```python
from build123d import *

# Parameters (mm, degrees)
BOSS_EXTRUDE1_DEPTH     = 15.24
SKETCH3_R               = 2.5
BOSS_EXTRUDE2_DEPTH     = 2.54
SKETCH4_W               = 6.457620629
SKETCH4_H               = 27.913585942
BOSS_EXTRUDE3_DEPTH     = 7.62
SKETCH11_W              = 6.457620629
SKETCH11_H              = 27.913585942
BOSS_EXTRUDE6_DEPTH     = 2.0955
CUT_EXTRUDE1_DEPTH      = 111.34392643
CUT_EXTRUDE1_DEPTH_BACK = 3.332
SKETCH6_R               = 2.15
FILLET1_R               = 0.508
SKETCH8_W               = 21.59
SKETCH8_H               = 20.32
CUT_EXTRUDE2_DEPTH      = 111.477226273
SKETCH1_3_W             = 10
SKETCH1_3_H             = 13.208
SKETCH1_3_R             = 2
BOSS_EXTRUDE5_DEPTH     = 2.54
CUT_EXTRUDE5_DEPTH      = 9.2075
CUT_EXTRUDE5_DEPTH_BACK = 117.302117887
SKETCH14_W              = 50.8
SKETCH14_H              = 3.81
BOSS_EXTRUDE7_START     = -7.62
SKETCH15_W              = 5.08
SKETCH15_H              = 5.08
SKETCH15_H_2            = 8.89
BOSS_EXTRUDE7_DEPTH     = 7.62
CUT_EXTRUDE6_REACH      = 118.302
SKETCH16_R              = 1.0922
SKETCH18_W              = 22.782868823
SKETCH18_H              = 5.08
BOSS_EXTRUDE8_DEPTH     = 5.08
CUT_EXTRUDE3_DEPTH      = 12.7
CUT_EXTRUDE3_DEPTH_BACK = 12.7
SKETCH9_R               = 1.4986
SKETCH10_R              = 2.794
CUT_EXTRUDE4_DEPTH      = 2
SKETCH20_R              = 2.15
BOSS_EXTRUDE9_DEPTH     = 1
BOSS_EXTRUDE10_START    = -1
SKETCH21_R              = 2.15
BOSS_EXTRUDE10_DEPTH    = 1


with BuildPart() as part:
    # Sketch1 → Boss-Extrude1 (new body)
    with BuildSketch(Plane(origin=(0, 0, 0), x_dir=(1, 0, 0), z_dir=(0, 1, 0))):
        Polygon((-58.867621619, 16.51), (-58.867621619, -16.51), (96.852680324, -16.51), (96.852680324, -11.43), (55.88, -11.43), (55.88, 8.89), (106.68, 8.89), (106.68, 16.51), align=None)
    extrude(amount=BOSS_EXTRUDE1_DEPTH)

    # Sketch3 → Boss-Extrude2 (add)
    with BuildSketch(Plane.XY.offset(16.51)):
        with BuildLine():
            Line((4.445, 15.24), (-4.445, 15.24))
            Line((-4.445, 15.24), (-4.445, 34.29))
            ThreePointArc((-4.445, 34.29), (0, 38.735), (4.445, 34.29))
            Line((4.445, 34.29), (4.445, 15.24))
        make_face()
        with Locations((0, 34.29)):
            Circle(SKETCH3_R, mode=Mode.SUBTRACT)
    boss_extrude2 = extrude(amount=-BOSS_EXTRUDE2_DEPTH)

    # Mirror1: Boss-Extrude2 across plane
    add(boss_extrude2.mirror(Plane.XY))

    # Sketch4 → Boss-Extrude3 (add)
    with BuildSketch(Plane(origin=(0, 15.24, 0), x_dir=(1, 0, 0), z_dir=(0, 1, 0))):
        with Locations((29.475913514, 0)):
            Rectangle(SKETCH4_W, SKETCH4_H)
        with Locations((-29.475913514, 0)):
            Rectangle(SKETCH4_W, SKETCH4_H)
    extrude(amount=BOSS_EXTRUDE3_DEPTH)

    # Sketch11 → Boss-Extrude6 (add)
    with BuildSketch(Plane(origin=(0, 22.86, 0), x_dir=(1, 0, 0), z_dir=(0, 1, 0))):
        with Locations((29.475913514, 0)):
            Rectangle(SKETCH11_W, SKETCH11_H)
    extrude(amount=BOSS_EXTRUDE6_DEPTH)

    # Sketch6 → Cut-Extrude1 (cut, two sides: drawn at the far end of the back side and taken through both)
    with BuildSketch(Plane(origin=(0, 22.86, 0), x_dir=(1, 0, 0), z_dir=(0, 1, 0)).offset(-CUT_EXTRUDE1_DEPTH_BACK)):
        with Locations(Location((29.5986053, 8.550450758, 0), (0, 0, 270))):
            Circle(SKETCH6_R)
        with Locations(Location((29.5986053, -8.550450758, 0), (0, 0, 270))):
            Circle(SKETCH6_R)
        with Locations(Location((-29.5986053, -8.550450758, 0), (0, 0, 90))):
            Circle(SKETCH6_R)
        with Locations(Location((-29.5986053, 8.550450758, 0), (0, 0, 90))):
            Circle(SKETCH6_R)
    extrude(amount=CUT_EXTRUDE1_DEPTH + CUT_EXTRUDE1_DEPTH_BACK, mode=Mode.SUBTRACT)

    # Fillet1
    fillet1_edges = [part.edges().sort_by_distance(p)[0] for p in [
        (-58.867621619, 0, 0),
        (106.68, 0, -12.7),
        (18.992529352, 0, 16.51),
        (-58.867621619, 7.62, 16.51),
        (-58.867621619, 7.62, -16.51),
        (106.68, 7.62, -16.51),
        (106.68, 7.62, -8.89),
        (96.852680324, 7.62, 16.51),
        (106.68, 15.24, -12.7),
        (-58.867621619, 15.24, 0),
        (-26.247103199, 22.86, 0),
        (-29.475913514, 22.86, -13.956792971),
        (-32.704723828, 22.86, 0),
        (-29.475913514, 22.86, 13.956792971),
        (32.704723828, 24.9555, 0),
        (29.475913514, 24.9555, -13.956792971),
        (26.247103199, 24.9555, 0),
        (29.475913514, 24.9555, 13.956792971),
    ]]
    fillet(fillet1_edges, radius=FILLET1_R)

    # Sketch8 → Cut-Extrude2 (cut, through all)
    with BuildSketch(Plane(origin=(0, 15.24, 0), x_dir=(1, 0, 0), z_dir=(0, 1, 0))):
        with Locations((46.028773367, -1.27)):
            Rectangle(SKETCH8_W, SKETCH8_H)
    extrude(amount=-CUT_EXTRUDE2_DEPTH, mode=Mode.SUBTRACT)

    # Sketch1<3> → Boss-Extrude5 (add)
    # profile 1 of 2: a face of its own
    with BuildSketch(Plane(origin=(0, 0, 0), x_dir=(1, 0, 0), z_dir=(0, 1, 0))):
        with Locations((-41.488351659, 23.114)):
            Rectangle(SKETCH1_3_W, SKETCH1_3_H)
        with Locations(Location((-41.488351659, 20.01, 0), (0, 0, 270))):
            Circle(SKETCH1_3_R, mode=Mode.SUBTRACT)
    # profile 2 of 2: a face of its own
    with BuildSketch(Plane(origin=(0, 0, 0), x_dir=(1, 0, 0), z_dir=(0, 1, 0))):
        with Locations((41.488351659, 23.114)):
            Rectangle(SKETCH1_3_W, SKETCH1_3_H)
        with Locations(Location((41.488351659, 20.01, 0), (0, 0, 270))):
            Circle(SKETCH1_3_R, mode=Mode.SUBTRACT)
    extrude(amount=BOSS_EXTRUDE5_DEPTH)

    # Sketch14 → Cut-Extrude5 (cut, two sides: drawn at the far end of the back side and taken through both)
    with BuildSketch(Plane.XY.offset(-8.89).offset(-CUT_EXTRUDE5_DEPTH_BACK)):
        with Locations((81.28, 13.335)):
            Rectangle(SKETCH14_W, SKETCH14_H)
    extrude(amount=CUT_EXTRUDE5_DEPTH + CUT_EXTRUDE5_DEPTH_BACK, mode=Mode.SUBTRACT)

    # Sketch15 → Boss-Extrude7 (add)
    with BuildSketch(Plane.XY.offset(-8.89).offset(BOSS_EXTRUDE7_START)):
        with Locations((53.34, 17.78)):
            Rectangle(SKETCH15_W, SKETCH15_H)
        with Locations((82.169, 15.875)):
            Rectangle(SKETCH15_W, SKETCH15_H_2)
    extrude(amount=BOSS_EXTRUDE7_DEPTH)

    # Sketch16 → Cut-Extrude6 (cut, up to next)
    with BuildSketch(Plane.XY.offset(-8.89), mode=Mode.PRIVATE) as cut_extrude6_sk1:
        with Locations((53.34, 17.526)):
            Circle(SKETCH16_R)
    cut_extrude6_tool1 = extrude(cut_extrude6_sk1.sketch, amount=-CUT_EXTRUDE6_REACH, mode=Mode.PRIVATE) & part.part
    # Sketch16 → Cut-Extrude6 (cut, up to next)
    with BuildSketch(Plane.XY.offset(-8.89), mode=Mode.PRIVATE) as cut_extrude6_sk2:
        with Locations((81.7245, 17.526)):
            Circle(SKETCH16_R)
    cut_extrude6_tool2 = extrude(cut_extrude6_sk2.sketch, amount=-CUT_EXTRUDE6_REACH, mode=Mode.PRIVATE) & part.part
    add(cut_extrude6_tool1.solids().sort_by_distance((53.34, 17.526, -8.89))[0], mode=Mode.SUBTRACT)
    add(cut_extrude6_tool2.solids().sort_by_distance((81.7245, 17.526, -8.89))[0], mode=Mode.SUBTRACT)

    # Sketch18 → Boss-Extrude8 (add)
    with BuildSketch(Plane(origin=(0, 15.24, 0), x_dir=(1, 0, 0), z_dir=(0, 1, 0))):
        with Locations((84.032315508, -13.97)):
            Rectangle(SKETCH18_W, SKETCH18_H)
    extrude(amount=BOSS_EXTRUDE8_DEPTH)

    # Sketch9 → Cut-Extrude3 (cut, two sides: drawn at the far end of the back side and taken through both)
    with BuildSketch(Plane(origin=(0, 0, 11.43), x_dir=(-1, 0, 0), z_dir=(0, 0, -1)).offset(-CUT_EXTRUDE3_DEPTH_BACK)):
        with Locations((-87.713434176, 16.836660264)):
            Circle(SKETCH9_R)
        with Locations((-78.658323849, 15.24)):
            Circle(SKETCH9_R)
    extrude(amount=CUT_EXTRUDE3_DEPTH + CUT_EXTRUDE3_DEPTH_BACK, mode=Mode.SUBTRACT)

    # Sketch10 → Cut-Extrude4 (cut)
    with BuildSketch(Plane.XY.offset(16.51)):
        with Locations((78.658323849, 15.24)):
            Circle(SKETCH10_R)
        with Locations((87.713434176, 16.836660264)):
            Circle(SKETCH10_R)
    extrude(amount=-CUT_EXTRUDE4_DEPTH, mode=Mode.SUBTRACT)

    # Sketch20 → Boss-Extrude9 (add)
    with BuildSketch(Plane(origin=(0, 22.86, 0), x_dir=(1, 0, 0), z_dir=(0, 1, 0))):
        with Locations(Location((-29.5986053, -8.550450758, 0), (0, 0, 270))):
            Circle(SKETCH20_R)
        with Locations(Location((-29.5986053, 8.550450758, 0), (0, 0, 270))):
            Circle(SKETCH20_R)
    extrude(amount=-BOSS_EXTRUDE9_DEPTH)

    # Sketch21 → Boss-Extrude10 (add)
    with BuildSketch(Plane(origin=(0, 24.9555, 0), x_dir=(1, 0, 0), z_dir=(0, 1, 0)).offset(BOSS_EXTRUDE10_START)):
        with Locations(Location((29.5986053, -8.550450758, 0), (0, 0, 270))):
            Circle(SKETCH21_R)
        with Locations(Location((29.5986053, 8.550450758, 0), (0, 0, 270))):
            Circle(SKETCH21_R)
    extrude(amount=BOSS_EXTRUDE10_DEPTH)


solid = part.part
```
Here's how the part is built. I have some questions about the finished solid (model axes, mm). A direction names the side the tool comes from. Give positions to 0.01 mm unless a question says otherwise; leave off trailing zeros. Order: outer loops, then holes, each group sorted by start corner. A loop starts at its lowest first (then second) coordinate and runs counter-clockwise, first axis right, second up. Notation, with made-up numbers: (20.5, 0) - (44.5, 0) arc R22 ccw to (44.5, 39) - close; hole circle Ø7 at (4.25, -23). An arc over 180 degrees is marked (long way). Answer as a JSON object with one key per item and string values. Group by question number.
Item 1: Which directions (+Z, -Z, +X, -X, +Y, -Y) give clear straight access to the entire face, cutting with the end or side of a thin tool? Please do faces 4 (the flat face through (84, 20.32, 14)), 5 (the flat face through (50.8, 18, -13)), 6 (the cylindrical face through (-31.052, 20.678, -6.966)), 7 (the flat face through (96.853, 8, 14)).
Item 2: For P1, Ø2.5, axis at x = -29.5, z = 3, coming from the +Y side; P2, Ø2.5, axis at x = 53, z = -13.5, coming from the +Y side; P3, Ø4, axis at x = 68.5, z = -15.5, coming from the +Y side, each with a flat end and sliding along its axis, tell me the tip position at first contact or that it passes through.
Item 3: If we section it at A-A on x = 48.5: Please give me the cut outline in (y, z), and give its area (3 significant figures).
Item 4: If we section it at D-D on z = 2: Please give me the cut outline in (x, y), and give its area (3 significant figures).
Item 5: If we section it at C-C on y = 6: Please give me the cut outline in (x, z).
Item 6: Please list where these lines run through material, in increasing order: probe 1 along X at (y, z) = (15.5, -15.5) (3 decimals); probe 2 along X at (y, z) = (1.6, -20.01); probe 3 along X at (y, z) = (34, 15) (3 decimals).
Item 7: If we section it at B-B on x = 0: Please give me the cut outline in (y, z) (3 decimals).
Item 8: If we mould it in two halves opening along Y, with no side actions, what happens to faces 1 (the cylindrical face through (-1, 32, -15)), 2 (the cylindrical face through (-0.098, 38.734, 15.258)), 3 (the flat face through (-26.247, 19, 0))? For each: pulls with the +Y half, pulls with the -Y half, needs draft (parallel to the pull), parting line crosses it, or undercut.
Result set:
{
 "1": {"face 4": "+Z, -Z, +X, +Y", "face 5": "+Z, -Z, +Y", "face 6": "none", "face 7": "+Z, +X, +Y, -Y"},
 "2": {"P1": "y = 22.86", "P2": "y = 20.32", "P3": "y = 11.43"},
 "3": {"outline": "(0, -16.51) - (15.24, -16.51) - (15.24, -8.89) - (0, -8.89) - close; (0, 11.43) - (15.24, 11.43) - (15.24, 16.51) - (0.51, 16.51) arc R0.51 ccw to (0, 16) - close", "area": "193 mm²"},
 "4": {"outline": "(-58.87, 0.51) arc R0.51 ccw to (-58.36, 0) - (35.23, 0) - (35.23, 15.24) - (32.7, 15.24) - (32.7, 24.45) arc R0.51 ccw to (32.2, 24.96) - (26.76, 24.96) arc R0.51 ccw to (26.25, 24.45) - (26.25, 15.24) - (-26.25, 15.24) - (-26.25, 22.35) arc R0.51 ccw to (-26.76, 22.86) - (-32.2, 22.86) arc R0.51 ccw to (-32.7, 22.35) - (-32.7, 15.24) - (-58.36, 15.24) arc R0.51 ccw to (-58.87, 14.73) - close", "area": "1,550 mm²"},
 "5": {"outline": "(-58.87, -16) arc R0.51 ccw to (-58.36, -16.51) - (106.17, -16.51) arc R0.51 ccw to (106.68, -16) - (106.68, -9.4) arc R0.51 ccw to (106.17, -8.89) - (35.23, -8.89) - (35.23, 11.43) - (96.85, 11.43) - (96.85, 16) arc R0.51 ccw to (96.34, 16.51) - (-58.36, 16.51) arc R0.51 ccw to (-58.87, 16) - close"},
 "6": {"probe 1": "-4.445 to 4.445, 50.8 to 55.88, 79.629 to 84.709", "probe 2": "-46.49 to -43.49, -39.49 to -36.49, 36.49 to 39.49, 43.49 to 46.49", "probe 3": "-4.445 to -2.483, 2.483 to 4.445"},
 "7": {"outline": "(0, -16.51) - (31.79, -16.51) - (31.79, -13.97) - (15.24, -13.97) - (15.24, 13.97) - (31.79, 13.97) - (31.79, 16.51) - (0.508, 16.51) arc R0.508 ccw to (0, 16.002) - close; (36.79, -16.51) - (38.735, -16.51) - (38.735, -13.97) - (36.79, -13.97) - close; (36.79, 13.97) - (38.735, 13.97) - (38.735, 16.51) - (36.79, 16.51) - close"},
 "8": {"face 1": "undercut", "face 2": "pulls with the +Y half", "face 3": "needs draft"}
}
